Geometry: final body of the model. Coordinates: model frame, mm. A direction names the side the tool comes from. Give positions to 0.01 mm unless a question says otherwise; leave off trailing zeros. Loops run counter-clockwise (first coordinate to the right, second up) from the corner with the lowest first, then second, coordinate; pieces in that order, holes last. Notation, with made-up numbers: M 82.5,17 L 107.5,17 A32 ccw 107.5,53 Z; hole C 30.25,-3.5 d3. An arc over 180 degrees is marked long. One line per question, with ' | ' between items. Start each with the question number.
from build123d import *

# Parameters (mm, degrees)
SKETCH3_R                       = 19.075
SKETCH3_R_2                     = 2.525
BOSS_EXTRUDE1_DEPTH             = 12.7
M5X0_8_TAPPED_HOLE1_D           = 4.2
M5X0_8_TAPPED_HOLE1_CSINK_D     = 5.05
M5X0_8_TAPPED_HOLE1_CSINK_ANGLE = 90
SKETCH8_R                       = 5.5
CUT_EXTRUDE1_DEPTH              = 7
BOSS_EXTRUDE2_DEPTH             = 12.7
FILLET1_R                       = 3
FILLET2_R                       = 3
CHAMFER1_SIZE                   = 1
M3X0_5_TAPPED_HOLE2_D           = 2.5


with BuildPart() as part:
    # Sketch3 → Boss-Extrude1 (new body)
    with BuildSketch(Plane.XY):
        Polygon((-50, 35.4), (50, 35.4), (50, 22.7), (30, -30), (-30, -30), (-50, 22.7), align=None)
        Circle(SKETCH3_R, mode=Mode.SUBTRACT)
        with Locations((-42, 29.05)):
            Circle(SKETCH3_R_2, mode=Mode.SUBTRACT)
        with Locations(Location((42, 29.05, 0), (0, 0, 180))):
            Circle(SKETCH3_R_2, mode=Mode.SUBTRACT)
        with Locations((-14, 29.05)):
            Circle(SKETCH3_R_2, mode=Mode.SUBTRACT)
        with Locations(Location((14, 29.05, 0), (0, 0, 180))):
            Circle(SKETCH3_R_2, mode=Mode.SUBTRACT)
    extrude(amount=-BOSS_EXTRUDE1_DEPTH)

    # M5x0.8 Tapped Hole1 (through all)
    with Locations(Plane.XY):
        with Locations((-25, 25), (25, 25), (25, -25), (-25, -25)):
            CounterSinkHole(M5X0_8_TAPPED_HOLE1_D / 2, M5X0_8_TAPPED_HOLE1_CSINK_D / 2, counter_sink_angle=M5X0_8_TAPPED_HOLE1_CSINK_ANGLE)

    # Sketch8 → Cut-Extrude1 (cut)
    with BuildSketch(Plane.XY):
        with Locations((-42, 29.05)):
            Circle(SKETCH8_R)
        with Locations((-14, 29.05)):
            Circle(SKETCH8_R)
        with Locations((14, 29.05)):
            Circle(SKETCH8_R)
        with Locations((42, 29.05)):
            Circle(SKETCH8_R)
    extrude(amount=-CUT_EXTRUDE1_DEPTH, mode=Mode.SUBTRACT)

    # Sketch9 → Boss-Extrude2 (add)
    with BuildSketch(Plane.XY):
        Polygon((-30, -30), (-30, -35.5), (-42, -35.5), (-42, 1.62), align=None)
    extrude(amount=-BOSS_EXTRUDE2_DEPTH)

    # Fillet1
    fillet1_edges = [part.edges().sort_by_distance(p)[0] for p in [
        (-30, -30, -6.35),
        (-42, 1.62, -6.35),
    ]]
    fillet(fillet1_edges, radius=FILLET1_R)

    # Fillet2
    fillet2_edges = [part.edges().sort_by_distance(p)[0] for p in [
        (-30, -35.5, -6.35),
    ]]
    fillet(fillet2_edges, radius=FILLET2_R)

    # Chamfer1
    chamfer1_edges = [part.edges().sort_by_distance(p)[0] for p in [
        (-42, -35.5, -6.35),
    ]]
    chamfer(chamfer1_edges, length=CHAMFER1_SIZE)

    # M3x0.5 Tapped Hole2 (through all)
    with Locations(Plane.XY):
        with Locations((-37, -13.5), (-37, -25.5)):
            Hole(M3X0_5_TAPPED_HOLE2_D / 2)


solid = part.part
Q1. Draft query along Y for faces 1 (the flat face through (2, -30, -6)), 2 (the flat face through (16.4, 30.3, -7)), 3 (the flat face through (-50, 29, -6)). Return one class per face: released by +Y, released by -Y, zero draft, split by the parting line, or undercut.
Q2. Section C-C, the plane y = 25. Count the separate pieces of the cut face and the enclosed holes in it, plus the area to 3 significant figures.
Q3. Section B-B, the plane x = 42. Output: boundary loops of the cut face in (y, z) (3 decimals), plus the area to 3 significant figures.
Q4. Contact query for flat-ended pins moving along their axis: pin 1 (4.5 mm diameter, centred on x = 42, y = 29.05, fed in from +Z); pin 2 (4 mm diameter, centred on x = -10, z = -3, fed in from -Y); pin 3 (4 mm diameter, centred on y = 13, z = -10.5, fed in from +X); pin 4 (5.5 mm diameter, centred on x = -12, y = 28.5, fed in from +Z). Output: stop coordinate, or through.
Q5. Section A-A, the plane x = -25. Output: boundary loops of the cut face in (y, z) (3 decimals).
Q6. Set-up query: faces 4 (the cylindrical face through (-15.86, 30.76, -9.81)), 5 (the cylindrical face through (16.957, 33.688, -3.451)). Return all of +Z, -Z, +X, -X, +Y, -Y with unobstructed straight access to the full face (end or side cutting, diameter ignored); none if empty.
Q7. Material intervals for L1, parallel to Y at x = 25, z = -5; L2, parallel to X at y = -24, z = -9; L3, parallel to X at y = -23.5, z = -8.5, sorted ascending.
Model answer:
1) face 1: released by -Y | face 2: undercut | face 3: zero draft
2) separate pieces: 3 | enclosed holes: 0 | area: 955 mm^2
3) outline: M 1.62,-12.7 L 26.525,-12.7 L 26.525,-7 L 23.55,-7 L 23.55,0 L 1.62,0 Z; M 31.575,-12.7 L 35.4,-12.7 L 35.4,0 L 34.55,0 L 34.55,-7 L 31.575,-7 Z | area: 323 mm^2
4) pin 1: passes through | pin 2: stops at y = -30 | pin 3: stops at x = 47.08 | pin 4: stops at z = -7
5) outline: M -30,-12.7 L -27.1,-12.7 L -27.1,-0.425 L -27.525,0 L -30,0 Z; M -22.9,-12.7 L 22.9,-12.7 L 22.9,-0.425 L 22.475,0 L -22.475,0 L -22.9,-0.425 Z; M 27.1,-12.7 L 35.4,-12.7 L 35.4,0 L 27.525,0 L 27.1,-0.425 Z
6) face 4: +Z, -Z | face 5: +Z
7) L1: y = -30 to -27.1, -22.9 to 22.9, 27.1 to 35.4 | L2: x = -42 to -26.85, -23.15 to 23.15, 26.85 to 32.28 | L3: x = -42 to -26.47, -23.53 to 23.53, 26.47 to 32.47
